The listing builds one solid part. Answer for the finished solid, in the listing's coordinates (mm). A direction names the side the tool comes from. Give positions to 0.01 mm unless a question says otherwise; leave off trailing zeros. Write each loop counter-clockwise with the first axis right and the second up, starting at its lowest first coordinate (ties: lowest second). Pieces come first, ordered by that corner, then holes. Notation, with made-up numbers: (25.25, 17) - (59.25, 17) arc R4 ccw to (59.25, 23) - close; hole circle Ø6 at (20, 19). An arc over 180 degrees is marked (long way). Return JSON: item names as keys, results as strings.
from build123d import *

# Parameters (mm, degrees)
SKETCH1_R                 = 0.725
BOSS_EXTRUDE1_DEPTH       = 2.54
SKETCH2_R                 = 1.651
BOSS_EXTRUDE2_DEPTH       = 4.7625
SKETCH3_W                 = 3.175
SKETCH3_H                 = 15
CUT_EXTRUDE1_DEPTH        = 16
FILLET1_R                 = 3.175
F_5_0MM_DOWEL_HOLE1_D     = 5
F_5_0MM_DOWEL_HOLE1_DEPTH = 20
F_5_0MM_DOWEL_HOLE1_TIP   = 1.502151548


with BuildPart() as part:
    # Sketch1 → Boss-Extrude1 (new body)
    with BuildSketch(Plane(origin=(0, 0, 0), x_dir=(1, 0, 0), z_dir=(0, 1, 0))):
        Polygon((-17.5, 0), (-17.5, 35), (-10.5, 35), (-10.5, 17.22), (10.5, 17.22), (10.5, 35), (17.5, 35), (17.5, 0), align=None)
        with Locations((-14, 32.46)):
            Circle(SKETCH1_R, mode=Mode.SUBTRACT)
        with Locations((-14, 18.96)):
            Circle(SKETCH1_R, mode=Mode.SUBTRACT)
        with Locations((14, 32.46)):
            Circle(SKETCH1_R, mode=Mode.SUBTRACT)
        with Locations((14, 18.96)):
            Circle(SKETCH1_R, mode=Mode.SUBTRACT)
    extrude(amount=BOSS_EXTRUDE1_DEPTH)

    # Sketch2 → Boss-Extrude2 (add, symmetric)
    with BuildSketch(Plane(origin=(0, 0, 0), x_dir=(0, 0, -1), z_dir=(1, 0, 0))):
        Polygon((15, 2.54), (7.5, 18.54), (0, 2.54), align=None)
        with Locations((7.5, 9.94)):
            Circle(SKETCH2_R, mode=Mode.SUBTRACT)
    extrude(amount=BOSS_EXTRUDE2_DEPTH, both=True)

    # Sketch3 → Cut-Extrude1 (cut)
    with BuildSketch(Plane(origin=(0, 2.54, 0), x_dir=(1, 0, 0), z_dir=(0, 1, 0))):
        with Locations((0, 7.5)):
            Rectangle(SKETCH3_W, SKETCH3_H)
    extrude(amount=CUT_EXTRUDE1_DEPTH, mode=Mode.SUBTRACT)

    # Fillet1
    fillet1_edges = [part.edges().sort_by_distance(p)[0] for p in [
        (3.175, 18.54, -7.5),
        (-3.175, 18.54, -7.5),
    ]]
    fillet(fillet1_edges, radius=FILLET1_R)

    # Ø5.0mm Dowel Hole1
    with Locations(Plane.ZY.offset(4.7625)):
        with Locations((-7.5, 9.94)):
            Hole(F_5_0MM_DOWEL_HOLE1_D / 2, depth=F_5_0MM_DOWEL_HOLE1_DEPTH)
            with Locations((0, 0, -(F_5_0MM_DOWEL_HOLE1_DEPTH + F_5_0MM_DOWEL_HOLE1_TIP / 2))):  # 118° drill point
                Cone(0, F_5_0MM_DOWEL_HOLE1_D / 2, F_5_0MM_DOWEL_HOLE1_TIP, mode=Mode.SUBTRACT)


solid = part.part
Item 1: The mould has two halves that part along Y. Classify faces 6 (the face through (-3.15, 12.05, -8.84)), 7 (the face through (0, 2.54, -14)), 8 (the face through (-4.762, 7, -7)): +Y half, -Y half, draft (parallel to the pull), parting line (faces both ways), or undercut.
Answer below:
{"face 6": "undercut", "face 7": "+Y half", "face 8": "draft"}
Item 2: For faces 1 (the face through (-13.7, 1.3, -31.8)), 2 (the face through (4.762, 7, -7)), 3 (the face through (-1.588, 7, -7)), 4 (the face through (3.2, 7.4, -12.72)), 5 (the face through (10.5, 1, -26)), determine the directions among +Z, -Z, +X, -X, +Y, -Y from which every point of the face is accessible in a straight line to the end or side of a thin tool.
Answer below:
{"face 1": "+Y, -Y", "face 2": "+Z, -Z, +X, +Y", "face 3": "+Z, -Z, +Y", "face 4": "-Z, +X, -X, +Y", "face 5": "-Z, +Y, -Y"}
Item 3: A cutting plane is placed at D-D on z = -26.5. Determine the outline of the cut face in (x, y).
Answer below:
{"outline": "(-17.5, 0) - (-10.5, 0) - (-10.5, 2.54) - (-17.5, 2.54) - close; (10.5, 0) - (17.5, 0) - (17.5, 2.54) - (10.5, 2.54) - close"}
Item 4: A cutting plane is placed at C-C on y = 3.5. Determine the outline of the cut face in (x, z), then the cut area to 3 significant figures.
Answer below:
{"outline": "(-4.76, -14.55) - (-1.59, -14.55) - (-1.59, -0.45) - (-4.76, -0.45) - close; (1.59, -14.55) - (4.76, -14.55) - (4.76, -0.45) - (1.59, -0.45) - close", "area": "89.5 mm²"}
Item 5: A cutting plane is placed at A-A on x = 14. Determine the outline of the cut face in (y, z) (3 decimals), then the cut area to 3 significant figures.
Answer below:
{"outline": "(0, -35) - (2.54, -35) - (2.54, -33.185) - (0, -33.185) - close; (0, -31.735) - (2.54, -31.735) - (2.54, -19.685) - (0, -19.685) - close; (0, -18.235) - (2.54, -18.235) - (2.54, 0) - (0, 0) - close", "area": "81.5 mm²"}
Item 6: Flat-ended cylindrical pins translate along their axes: P1, Ø12, axis at x = 2.5, z = -19.5, coming from the +Y side; P2, Ø1.5, axis at x = -4.5, y = 9.5, coming from the +Z side; P3, Ø4, axis at x = -1, y = 5, coming from the +Z side. Find the tip coordinate at first contact, or state that the pin passes through.
Answer below:
{"P1": "stops at y = 5.74", "P2": "stops at z = -2.91", "P3": "stops at z = -0.26"}
Item 7: Consider L1, parallel to Z at x = 14, y = 0.7 (3 decimals); L2, parallel to X at y = 1.85, z = -32.46 (3 decimals); L3, parallel to X at y = 6.25, z = -5. Determine where each line is inside the solid, lowest interval first.
Answer below:
{"L1": "z = -35 to -33.185, -31.735 to -19.685, -18.235 to 0", "L2": "x = -17.5 to -14.725, -13.275 to -10.5, 10.5 to 13.275, 14.725 to 17.5", "L3": "x = -4.76 to -1.59, 1.59 to 4.76"}
Item 8: A cutting plane is placed at B-B on z = -18.96. Determine the outline of the cut face in (x, y) (3 decimals), then the cut area to 3 significant figures.
Answer below:
{"outline": "(-17.5, 0) - (-14.725, 0) - (-14.725, 2.54) - (-17.5, 2.54) - close; (-13.275, 0) - (-10.5, 0) - (-10.5, 2.54) - (-13.275, 2.54) - close; (10.5, 0) - (13.275, 0) - (13.275, 2.54) - (10.5, 2.54) - close; (14.725, 0) - (17.5, 0) - (17.5, 2.54) - (14.725, 2.54) - close", "area": "28.2 mm²"}
